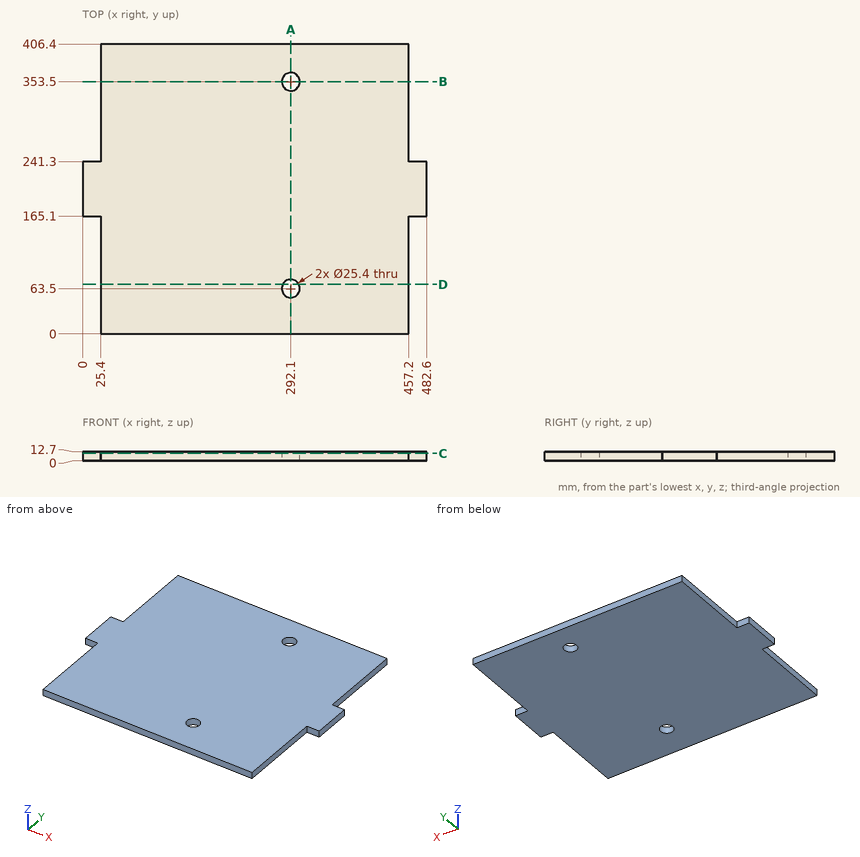
Geometry: see drawing. Coordinates: mm, zero at the bounding-box minimum. Coordinates: 2 decimals unless noted, no trailing zeros. Loops run counter-clockwise (first coordinate to the right, second up) from the corner with the lowest first, then second, coordinate; pieces in that order, holes last.
Q1. Cut plane D-D (y = 69.5). Output: boundary loops of the cut face in (x, z), then the cut area to 3 significant figures.
Q2. Cut plane B-B (y = 353.5). Output: boundary loops of the cut face in (x, z).
Q3. Cut plane C-C (z = 10.5). Output: boundary loops of the cut face in (x, y).
Q4. Contact query for flat-ended pins moving along their axis: pin 1 (6.5 mm diameter, centred on x = 464.5, z = 4.5, fed in from +Y); pin 2 (6.5 mm diameter, centred on y = 94.5, z = 5, fed in from +X); pin 3 (4 mm diameter, centred on y = 324, z = 4, fed in from -X). Output: stop coordinate, or through.
Q5. Cut plane A-A (x = 292.1). Output: boundary loops of the cut face in (y, z), then the cut area to 3 significant figures.
Q6. Material intervals for line 1 (Y direction, x = 292.1, z = 5.5); line 2 (X direction, y = 31, z = 5.5); line 3 (X direction, y = 58, z = 3.75), sorted ascending.
Working result:
1. outline: (25.4, 0) - (280.91, 0) - (280.91, 12.7) - (25.4, 12.7) - close; (303.29, 0) - (457.2, 0) - (457.2, 12.7) - (303.29, 12.7) - close
1. area: 5,200 mm2
2. outline: (25.4, 0) - (279.4, 0) - (279.4, 12.7) - (25.4, 12.7) - close; (304.8, 0) - (457.2, 0) - (457.2, 12.7) - (304.8, 12.7) - close
3. outline: (0, 165.1) - (25.4, 165.1) - (25.4, 0) - (457.2, 0) - (457.2, 165.1) - (482.6, 165.1) - (482.6, 241.3) - (457.2, 241.3) - (457.2, 406.4) - (25.4, 406.4) - (25.4, 241.3) - (0, 241.3) - close; hole circle Ø25.4 at (292.1, 63.5); hole circle Ø25.4 at (292.1, 353.5)
4. pin 1: stops at y = 241.3
4. pin 2: stops at x = 457.2
4. pin 3: stops at x = 25.4
5. outline: (0, 0) - (50.8, 0) - (50.8, 12.7) - (0, 12.7) - close; (76.2, 0) - (340.8, 0) - (340.8, 12.7) - (76.2, 12.7) - close; (366.2, 0) - (406.4, 0) - (406.4, 12.7) - (366.2, 12.7) - close
5. area: 4,520 mm2
6. line 1: y = 0 to 50.8, 76.2 to 340.8, 366.2 to 406.4
6. line 2: x = 25.4 to 457.2
6. line 3: x = 25.4 to 280.65, 303.55 to 457.2
